```python
from build123d import *

# Parameters (mm, degrees)
ESQUISSE1_R             = 1
ESQUISSE1_R_2           = 1.5
BOSS_EXTRU_1_DEPTH      = 5
ENL_V_MAT_EXTRU_1_DEPTH = 5
ESQUISSE3_W             = 20
ESQUISSE3_H             = 34
BOSS_EXTRU_2_DEPTH      = 5
ESQUISSE4_R             = 1.5
ESQUISSE4_W             = 9.798464728
ESQUISSE4_H             = 39.858161606
ENL_V_MAT_EXTRU_2_DEPTH = 5
ESQUISSE5_W             = 2.5
ESQUISSE5_H             = 34
BOSS_EXTRU_3_DEPTH      = 5
ESQUISSE6_R             = 1.6
BOSS_EXTRU_4_DEPTH      = 5
ESQUISSE8_W             = 43.131619687
ESQUISSE8_H             = 48.78573065
ESQUISSE8_W_2           = 13.204377845
ESQUISSE8_H_2           = 47.447309867
ENL_V_MAT_EXTRU_3_DEPTH = 10
ESQUISSE9_R             = 1.5
ESQUISSE9_R_2           = 1
BOSS_EXTRU_5_DEPTH      = 5
CONG_1_R                = 10


with BuildPart() as part:
    # Esquisse1 → Boss.-Extru.1 (new body)
    with BuildSketch(Plane.XY):
        with BuildLine():
            Line((-13.584596858, -30.047129187), (-13.584596858, -25.547129187))
            Line((-13.584596858, -25.547129187), (-13.584596858, -25.297129187))
            Line((-13.584596858, -25.297129187), (-13.834596858, -25.297129187))
            Line((-13.834596858, -25.297129187), (-16.334596858, -25.297129187))
            Line((-16.334596858, -25.297129187), (-16.584596858, -25.297129187))
            Line((-16.584596858, -25.297129187), (-16.584596858, -25.047129187))
            Line((-16.584596858, -25.047129187), (-16.584596858, 6.452870813))
            Line((-16.584596858, 6.452870813), (-16.584596858, 6.702870813))
            Line((-16.584596858, 6.702870813), (-16.334596858, 6.702870813))
            Line((-16.334596858, 6.702870813), (-13.834596858, 6.702870813))
            Line((-13.834596858, 6.702870813), (-13.584596858, 6.702870813))
            Line((-13.584596858, 6.702870813), (-13.584596858, 6.952870813))
            Line((-13.584596858, 6.952870813), (-13.584596858, 11.452870813))
            Line((-13.584596858, 11.452870813), (-13.584596858, 11.702870813))
            Line((-13.584596858, 11.702870813), (-13.334596858, 11.702870813))
            Line((-13.334596858, 11.702870813), (-8.584596858, 11.702870813))
            Line((-8.584596858, 11.702870813), (-8.584596858, 6.702870813))
            Line((-8.584596858, 6.702870813), (-7.491776281, 6.702870813))
            Line((-7.491776281, 6.702870813), (-4.034541178, 6.702870813))
            ThreePointArc((-4.034541178, 6.702870813), (-0.161557832, 6.19424756), (3.448773595, 4.702870813))
            ThreePointArc((3.448773595, 4.702870813), (10.66943645, 1.720117321), (18.415403142, 0.702870813))
            ThreePointArc((18.415403142, 0.702870813), (28.415403142, -9.297129187), (18.415403142, -19.297129187))
            ThreePointArc((18.415403142, -19.297129187), (10.66943645, -20.314375694), (3.448773595, -23.297129187))
            ThreePointArc((3.448773595, -23.297129187), (-0.161557832, -24.788505933), (-4.034541178, -25.297129187))
            Line((-4.034541178, -25.297129187), (-7.491776281, -25.297129187))
            Line((-7.491776281, -25.297129187), (-8.584596858, -25.297129187))
            Line((-8.584596858, -25.297129187), (-8.584596858, -30.297129187))
            Line((-8.584596858, -30.297129187), (-13.334596858, -30.297129187))
            Line((-13.334596858, -30.297129187), (-13.584596858, -30.297129187))
            Line((-13.584596858, -30.297129187), (-13.584596858, -30.047129187))
        make_face()
        with Locations((18.477857718, -2.297129187)):
            Circle(ESQUISSE1_R, mode=Mode.SUBTRACT)
        with Locations((25.415403142, -9.359583762)):
            Circle(ESQUISSE1_R, mode=Mode.SUBTRACT)
        with Locations((18.415403142, -9.297129187)):
            Circle(ESQUISSE1_R_2, mode=Mode.SUBTRACT)
        with Locations((11.415403142, -9.234674611)):
            Circle(ESQUISSE1_R, mode=Mode.SUBTRACT)
        with Locations((18.352948567, -16.297129187)):
            Circle(ESQUISSE1_R, mode=Mode.SUBTRACT)
    extrude(amount=BOSS_EXTRU_1_DEPTH)

    # Esquisse2 → Enlèv. mat.-Extru.1 (cut)
    with BuildSketch(Plane(origin=(0, 0, 0), x_dir=(-1, 0, 0), z_dir=(0, 0, -1))):
        Polygon((1.584596858, -19.297129187), (1.584596858, -25.297129187), (1.584596858, -26.297129187), (21.584596858, -26.297129187), (21.584596858, -33.65697819), (-26.833247513, -33.65697819), (-26.198667142, -19.297129187), align=None)
        Polygon((21.584596858, 7.702870813), (1.584596858, 7.702870813), (1.584596858, 6.702870813), (1.584596858, 0.702870813), (-26.198667142, 0.702870813), (-26.833247513, 15.062719816), (21.584596858, 15.062719816), align=None)
    extrude(amount=-ENL_V_MAT_EXTRU_1_DEPTH, mode=Mode.SUBTRACT)

    # Esquisse3 → Boss.-Extru.2 (add)
    with BuildSketch(Plane(origin=(0, 0, 0), x_dir=(-1, 0, 0), z_dir=(0, 0, -1))):
        with Locations((11.584596858, -9.297129187)):
            Rectangle(ESQUISSE3_W, ESQUISSE3_H)
    extrude(amount=-BOSS_EXTRU_2_DEPTH)

    # Esquisse4 → Enlèv. mat.-Extru.2 (cut)
    with BuildSketch(Plane(origin=(0, 0, 0), x_dir=(-1, 0, 0), z_dir=(0, 0, -1))):
        with Locations((9.084596858, -22.797129187)):
            Circle(ESQUISSE4_R)
        with Locations((9.084596858, 4.202870813)):
            Circle(ESQUISSE4_R)
        with Locations((23.983829222, -9.020336398)):
            Rectangle(ESQUISSE4_W, ESQUISSE4_H)
    extrude(amount=-ENL_V_MAT_EXTRU_2_DEPTH, mode=Mode.SUBTRACT)

    # Esquisse5 → Boss.-Extru.3 (add)
    with BuildSketch(Plane(origin=(0, 0, 0), x_dir=(-1, 0, 0), z_dir=(0, 0, -1))):
        with Locations((0.334596858, -9.297129187)):
            Rectangle(ESQUISSE5_W, ESQUISSE5_H)
    extrude(amount=-BOSS_EXTRU_3_DEPTH)

    # Esquisse6 → Boss.-Extru.4 (add)
    # profile 1 of 2: a face of its own
    with BuildSketch(Plane(origin=(0, 0, 0), x_dir=(-1, 0, 0), z_dir=(0, 0, -1))):
        with BuildLine():
            Line((12.324596858, -25.12480516), (5.844596858, -25.12480516))
            Line((5.844596858, -25.12480516), (5.844596858, -28.797129187))
            ThreePointArc((5.844596858, -28.797129187), (9.084596858, -32.037129187), (12.324596858, -28.797129187))
            Line((12.324596858, -28.797129187), (12.324596858, -25.12480516))
        make_face()
        with Locations((9.084596858, -28.797129187)):
            Circle(ESQUISSE6_R, mode=Mode.SUBTRACT)
    # profile 2 of 2: a face of its own
    with BuildSketch(Plane(origin=(0, 0, 0), x_dir=(-1, 0, 0), z_dir=(0, 0, -1))):
        with BuildLine():
            Line((12.324596858, 6.757738308), (5.844596858, 6.757738308))
            Line((5.844596858, 6.757738308), (5.844596858, 10.202870813))
            ThreePointArc((5.844596858, 10.202870813), (9.084596858, 13.442870813), (12.324596858, 10.202870813))
            Line((12.324596858, 10.202870813), (12.324596858, 6.757738308))
        make_face()
        with Locations((9.084596858, 10.202870813)):
            Circle(ESQUISSE6_R, mode=Mode.SUBTRACT)
    extrude(amount=-BOSS_EXTRU_4_DEPTH)

    # Esquisse8 → Enlèv. mat.-Extru.3 (cut)
    with BuildSketch(Plane(origin=(0, 0, 0), x_dir=(-1, 0, 0), z_dir=(0, 0, -1))):
        with Locations((-19.981212986, -14.067924119)):
            Rectangle(ESQUISSE8_W, ESQUISSE8_H)
        with Locations((23.186785781, -15.322061454)):
            Rectangle(ESQUISSE8_W_2, ESQUISSE8_H_2)
    extrude(amount=-ENL_V_MAT_EXTRU_3_DEPTH, mode=Mode.SUBTRACT)

    # Esquisse9 → Boss.-Extru.5 (add)
    with BuildSketch(Plane(origin=(0, 0, 0), x_dir=(-1, 0, 0), z_dir=(0, 0, -1))):
        with BuildLine():
            Line((-15.415403142, -19.297129187), (1.584596858, -19.297129187))
            Line((1.584596858, -19.297129187), (1.584596858, 0.702870813))
            Line((1.584596858, 0.702870813), (-15.415403142, 0.702870813))
            ThreePointArc((-15.415403142, 0.702870813), (-25.415403142, -9.297129187), (-15.415403142, -19.297129187))
        make_face()
        with Locations((-15.415403142, -9.297129187)):
            Circle(ESQUISSE9_R, mode=Mode.SUBTRACT)
        with Locations((-15.415403142, -15.934238111)):
            Circle(ESQUISSE9_R_2, mode=Mode.SUBTRACT)
        with Locations((-22.758101932, -9.297129187)):
            Circle(ESQUISSE9_R_2, mode=Mode.SUBTRACT)
        with Locations((-15.415403142, -3.255710211)):
            Circle(ESQUISSE9_R_2, mode=Mode.SUBTRACT)
        with Locations((-7.938498128, -9.297129187)):
            Circle(ESQUISSE9_R_2, mode=Mode.SUBTRACT)
    extrude(amount=-BOSS_EXTRU_5_DEPTH)

    # Congé1
    # the kernel refuses this fillet: 10 mm, written as the material it adds along each edge
    with BuildSketch(Plane(origin=(-1.584596858, 0.702870813, 0), x_dir=(0, 1, 0), z_dir=(0, 0, 1))) as cong_1_piece_1:
        with BuildLine():
            CenterArc((10, -9.539392014), CONG_1_R, 107.457603124, 72.542396876)
            Line((0, -9.539392014), (-0.2, -9.539392014))
            Line((-0.2, -9.539392014), (-0.2, 0))
            Line((-0.2, 0), (0, 0.2))
            ThreePointArc((0, 0.2), (3.5, 0.2), (6.94, 0.19078784))
            Line((6.94, 0.19078784), (7, 0))
        make_face()
    extrude(amount=5)
    with BuildSketch(Plane(origin=(-1.584596858, -19.297129187, 0), x_dir=(0, -1, 0), z_dir=(0, 0, 1))) as cong_1_piece_2:
        with BuildLine():
            CenterArc((10, 9.539392014), CONG_1_R, 180, 72.542396876)
            Line((0, 9.539392014), (-0.2, 9.539392014))
            Line((-0.2, 9.539392014), (-0.2, 0))
            Line((-0.2, 0), (0, -0.2))
            ThreePointArc((0, -0.2), (3.5, -0.2), (6.94, -0.19078784))
            Line((6.94, -0.19078784), (7, 0))
        make_face()
    extrude(amount=5)


solid = part.part
```
Here's how the part is built. I have some questions about the finished solid (model axes, mm). A direction names the side the tool comes from. Coordinates: 2 decimals unless noted, no trailing zeros. Order: outer loops, then holes, each group sorted by start corner. A loop starts at its lowest first (then second) coordinate and runs counter-clockwise, first axis right, second up.
1) Imagine slicing it at D-D on y = -17.5. List the corners of the cut face in (x, z) for me, and give its area (3 significant figures).
2) Imagine slicing it at B-B on x = -9.5. List the corners of the cut face in (y, z) for me, and give its area (3 significant figures).
3) I need wall thicknesses on line 1 (Y direction, x = 8, z = 2.1); line 2 (Y direction, x = 9, z = 2.2); line 3 (X direction, y = 8, z = 1.2). Which ranges of each line are inside material? Lowest first, please.
4) Imagine slicing it at A-A on z = 3.95. State how many separate pieces and enclosed holes the cut face has, and give its area (3 significant figures).
5) Imagine slicing it at C-C on x = -2.5. List the corners of the cut face in (y, z) for me.
6) Will these pins go through, and if not, where does the flat tip stop? pin 1 (4 mm diameter, centred on x = -3, y = -2.5, fed in from -Z); pin 2 (1.3 mm diameter, centred on y = 9, z = 1.5, fed in from -X); pin 3 (3 mm diameter, centred on y = -27.5, z = 3, fed in from +X).
7) Which directions (+Z, -Z, +X, -X, +Y, -Y) give clear straight access to the entire face, cutting with the end or side of a thin tool? Please do faces 1 (the face through (-14, -26.297, 2)), 2 (the face through (-14, 7.703, 2)), 3 (the face through (-4, -26.297, 2)).
8) We'd pull the mould along Y, two halves only. Please class faces 4 (the face through (-9.013, 13.442, 2.465)), 5 (the face through (-9.82, -30.22, 2.46)), 6 (the face through (12, -19.297, 2)), 7 (the face through (-5.845, -28, 2)): +Y half, -Y half, draft (parallel to the pull), parting line (faces both ways), or undercut.
Response values:
1. outline: (-16.58, 0) - (21.13, 0) - (21.13, 5) - (-16.58, 5) - close
1. area: 189 mm2
2. outline: (-32.01, 0) - (-30.34, 0) - (-30.34, 5) - (-32.01, 5) - close; (-27.25, 0) - (-24.24, 0) - (-24.24, 5) - (-27.25, 5) - close; (-21.36, 0) - (2.76, 0) - (2.76, 5) - (-21.36, 5) - close; (5.64, 0) - (8.66, 0) - (8.66, 5) - (5.64, 5) - close; (11.75, 0) - (13.42, 0) - (13.42, 5) - (11.75, 5) - close
2. area: 167 mm2
3. line 1: y = -19.3 to -10.3, -8.3 to 0.7
3. line 2: y = -19.3 to 0.7
3. line 3: x = -12.32 to -5.84
4. separate pieces: 1
4. enclosed holes: 9
4. area: 1,060 mm2
5. outline: (-26.3, 0) - (7.7, 0) - (7.7, 5) - (-26.3, 5) - close
6. pin 1: stops at z = 0
6. pin 2: stops at x = -12.32
6. pin 3: stops at x = -1.49
7. face 1: +Z, -Z, -X, -Y
7. face 2: +Z, -Z, -X, +Y
7. face 3: +Z, -Z, +X, -Y
8. face 4: +Y half
8. face 5: undercut
8. face 6: -Y half
8. face 7: draft
